Can you work these out from the model? Positions are in its coordinate system, mm. A direction names the side the tool comes from. Coordinates: 2 decimals unless noted, no trailing zeros. Loops run counter-clockwise (first coordinate to the right, second up) from the corner with the lowest first, then second, coordinate; pieces in that order, holes last. Notation, with made-up numbers: (74.5, -1) -> (97.5, -1) arc R29 cw to (97.5, 22) -> close; hole circle Ø6 at (62, 13). An arc over 180 degrees is marked (long way). Use one line per item in the form item = value. Start each with the question number.
(1) Imagine slicing it at B-B (y = 5.5). List the corners of the cut face in (x, z) for me.
(2) I need wall thicknesses on line 1 (Y direction, x = 1.4, z = 2.1); line 2 (Z direction, x = 9, y = 5.25); line 3 (X direction, y = 1, z = 3.1). Which ranges of each line are inside material? Lowest first, please. Write a range as [from, to].
(3) I'm going to push flat-ended pins straight in: pin 1 (0.8 mm diameter, centred on x = -2.5, z = 1.5, fed in from -Y); pin 2 (0.7 mm diameter, centred on x = 8.5, z = 1.5, fed in from +Y); pin 3 (0.8 mm diameter, centred on x = -2, y = 1, fed in from -Z). Where does each tip first touch, or does it pass through?
(4) On a 3-axis mill with a long thin cutter (end or side, diameter ignored), from which of +Z, -Z, +X, -X, +Y, -Y can I reach the whole of each face in a straight line? I mean faces 1 (the cylindrical face through (4.56, 0.76, 3.4)), 2 (the flat face through (-4, 2.6, 2.7)), 3 (the flat face through (-1, 3, 1.85)). Say none if no direction works.
(5) Thinking about a two-plate mould opening in X: for faces 4 (the flat face through (-4, 1.4, 1.5)), 5 (the flat face through (9, 1.4, 2)), 6 (the cylindrical face through (7.063, 2.954, 2.4)), which applies, released by +X, released by -X, zero draft, split by the parting line, or undercut?
(6) Imagine slicing it at D-D (y = 4.25). List the corners of the cut face in (x, z) for me, plus the area to 3 significant figures.
(7) Imagine slicing it at A-A (x = -0.5). List the corners of the cut face in (y, z) for me, plus the area to 3 significant figures.
(8) Imagine slicing it at C-C (x = 4.5). List the corners of the cut face in (y, z) for me, plus the area to 3 significant figures.
```python
from build123d import *
from build123d.topology import SkipClean

# Parameters (mm, degrees)
SKETCH_1_W          = 11.5
SKETCH_1_H          = 6
EXTRUDE_1_DEPTH     = 4.2
SKETCH_2_R          = 1.5
CUT_EXTRUDE_1_DEPTH = 2
SKETCH_3_R          = 1.3
EXTRUDE_2_DEPTH     = 6
CHAMFER_1_SIZE      = 0.2
CUT_EXTRUDE_START   = -5
CUT_EXTRUDE_2_DEPTH = 5
SKETCH_5_R          = 1
CUT_EXTRUDE_3_DEPTH = 9
SKETCH_6_R          = 1.3
CUT_EXTRUDE_4_DEPTH = 2
SKETCH_7_R          = 1.5
CUT_EXTRUDE_5_DEPTH = 1
CUT_EXTRUDE_6_DEPTH = 0.5
EXTRUDE_START       = -3
SKETCH_9_R          = 0.7
EXTRUDE_3_DEPTH     = 1.6
FILLET_1_R          = 0.2


with BuildPart() as part:
    # Sketch 1 → Extrude 1 (new body)
    with BuildSketch(Plane.XY):
        with Locations((5.75, 3)):
            Rectangle(SKETCH_1_W, SKETCH_1_H)
    extrude(amount=EXTRUDE_1_DEPTH)

    # Sketch 2 → Cut-Extrude 1 (cut)
    with BuildSketch(Plane.ZY):
        with Locations((2.1, 2)):
            Circle(SKETCH_2_R)
    extrude(amount=-CUT_EXTRUDE_1_DEPTH, mode=Mode.SUBTRACT)

    # Sketch 3 → Extrude 2 (add)
    with BuildSketch(Plane.ZY.offset(-2)):
        with Locations((2.1, 2)):
            Circle(SKETCH_3_R)
    extrude(amount=EXTRUDE_2_DEPTH)

    # Chamfer 1
    chamfer_1_edges = [part.edges().sort_by_distance(p)[0] for p in [
        (-4, 2, 0.8),
    ]]
    chamfer(chamfer_1_edges, length=CHAMFER_1_SIZE)

    # Sketch 4 → Cut-Extrude 2 (cut)
    with BuildSketch(Plane.ZY.offset(4).offset(CUT_EXTRUDE_START)):
        with BuildLine():
            Line((1.85, 3.275735082), (1.85, 2.25))
            Line((1.85, 2.25), (0.824264918, 2.25))
            ThreePointArc((0.824264918, 2.25), (0.8, 2), (0.824264918, 1.75))
            Line((0.824264918, 1.75), (1.85, 1.75))
            Line((1.85, 1.75), (1.85, 0.724264918))
            ThreePointArc((1.85, 0.724264918), (2.1, 0.7), (2.35, 0.724264918))
            Line((2.35, 0.724264918), (2.35, 1.75))
            Line((2.35, 1.75), (3.375735082, 1.75))
            ThreePointArc((3.375735082, 1.75), (3.4, 2), (3.375735082, 2.25))
            Line((3.375735082, 2.25), (2.35, 2.25))
            Line((2.35, 2.25), (2.35, 3.275735082))
            ThreePointArc((2.35, 3.275735082), (2.1, 3.3), (1.85, 3.275735082))
        make_face()
    extrude(amount=CUT_EXTRUDE_2_DEPTH, mode=Mode.SUBTRACT)

    # Sketch 5 → Cut-Extrude 3 (cut)
    with BuildSketch(Plane(origin=(11.5, 0, 0), x_dir=(0, 0, -1), z_dir=(1, 0, 0))):
        with Locations(Location((-2.1, 2, 0), (0, 0, 90))):
            Circle(SKETCH_5_R)
    extrude(amount=-CUT_EXTRUDE_3_DEPTH, mode=Mode.SUBTRACT)

    # Sketch 6 → Cut-Extrude 4 (cut)
    with BuildSketch(Plane.XZ):
        with Locations(Location((4.5, 2.1, 0), (0, 0, 270))):
            Circle(SKETCH_6_R)
    extrude(amount=-CUT_EXTRUDE_4_DEPTH, mode=Mode.SUBTRACT)

    # Sketch 7 → Cut-Extrude 5 (cut)
    with BuildSketch(Plane(origin=(0, 6, 0), x_dir=(1, 0, 0), z_dir=(0, 1, 0))):
        with Locations(Location((9, -2.1, 0), (0, 0, 270))):
            Circle(SKETCH_7_R)
    extrude(amount=-CUT_EXTRUDE_5_DEPTH, mode=Mode.SUBTRACT)

    # Sketch 8 → Cut-Extrude 6 (cut)
    with SkipClean():  # the faces are left unmerged after this step: merging them gives an invalid solid
        with BuildSketch(Plane(origin=(0, 5, 0), x_dir=(1, 0, 0), z_dir=(0, 1, 0))):
            with BuildLine():
                Line((9.088388348, -2.188388348), (8.03141744, -3.245359255))
                ThreePointArc((8.03141744, -3.245359255), (7.939339828, -3.160660172), (7.854640745, -3.06858256))
                Line((7.854640745, -3.06858256), (8.911611652, -2.011611652))
                Line((8.911611652, -2.011611652), (9.96858256, -0.954640745))
                ThreePointArc((9.96858256, -0.954640745), (10.060660172, -1.039339828), (10.145359255, -1.13141744))
                Line((10.145359255, -1.13141744), (9.088388348, -2.188388348))
            make_face()
        extrude(amount=-CUT_EXTRUDE_6_DEPTH, mode=Mode.SUBTRACT)

    # Sketch 9 → Extrude 3 (add)
    with SkipClean():  # the faces are left unmerged after this step: merging them gives an invalid solid
        with BuildSketch(Plane(origin=(0, 6, 0), x_dir=(1, 0, 0), z_dir=(0, 1, 0)).offset(EXTRUDE_START)):
            with Locations(Location((9, -2.1, 0), (0, 0, 270))):
                Circle(SKETCH_9_R)
        extrude(amount=-EXTRUDE_3_DEPTH)

    # Fillet 1
    fillet_1_edges = [part.edges().sort_by_distance(p)[0] for p in [
        (11.5, 3, 4.2),
        (5.75, 6, 4.2),
        (0, 3, 4.2),
        (5.75, 6, 0),
        (11.5, 3, 0),
        (5.75, 0, 0),
        (0, 3, 0),
        (5.75, 0, 4.2),
        (0, 6, 2.1),
        (11.5, 6, 2.1),
        (11.5, 0, 2.1),
        (0, 0, 2.1),
    ]]
    fillet(fillet_1_edges, radius=FILLET_1_R)


solid = part.part
```
Worked out:
q1.outline = (0, 0.2) arc R0.2 ccw to (0.2, 0) -> (11.3, 0) arc R0.2 ccw to (11.5, 0.2) -> (11.5, 4) arc R0.2 ccw to (11.3, 4.2) -> (0.2, 4.2) arc R0.2 ccw to (0, 4) -> close; hole circle Ø3 at (9, 2.1)
q2.line_1 = [0, 0.5], [0.7, 3.3], [3.5, 6]
q2.line_2 = [0, 0.6], [3.6, 4.2]
q2.line_3 = [2, 3.67], [5.33, 11.5]
q3.pin_1 = 0.72
q3.pin_2 = 5
q3.pin_3 = 0.95
q4.face_1 = -Y
q4.face_2 = +Z, -Z, -X, +Y, -Y
q4.face_3 = -X
q5.face_4 = released by -X
q5.face_5 = zero draft
q5.face_6 = undercut
q6.outline = (0, 0.2) arc R0.2 ccw to (0.2, 0) -> (11.3, 0) arc R0.2 ccw to (11.5, 0.2) -> (11.5, 4) arc R0.2 ccw to (11.3, 4.2) -> (0.2, 4.2) arc R0.2 ccw to (0, 4) -> close
q6.area = 48.3 mm2
q7.outline = (0.72, 1.85) arc R1.3 ccw to (1.75, 0.82) -> (1.75, 1.85) -> close; (0.72, 2.35) -> (1.75, 2.35) -> (1.75, 3.38) arc R1.3 ccw to start; (2.25, 0.82) arc R1.3 ccw to (3.28, 1.85) -> (2.25, 1.85) -> close; (2.25, 2.35) -> (3.28, 2.35) arc R1.3 ccw to (2.25, 3.38) -> close
q7.area = 2.98 mm2
q8.outline = (0, 0.2) arc R0.2 ccw to (0.2, 0) -> (5.8, 0) arc R0.2 ccw to (6, 0.2) -> (6, 4) arc R0.2 ccw to (5.8, 4.2) -> (0.2, 4.2) arc R0.2 ccw to (0, 4) -> (0, 3.4) -> (2, 3.4) -> (2, 3.1) arc R1 cw to (2, 1.1) -> (2, 0.8) -> (0, 0.8) -> close
q8.area = 18.4 mm2
